CAD build for the part. Positions are in the model's coordinates, mm. A direction names the side the tool comes from. Give positions to 0.01 mm unless a question says otherwise; leave off trailing zeros. Write each loop counter-clockwise with the first axis right and the second up, starting at its lowest first coordinate (ties: lowest second). Pieces come first, ordered by that corner, then holes. Notation, with made-up numbers: (47, 58.5) -> (67, 58.5) arc R22 ccw to (67, 93.5) -> close; hole circle Ø4 at (-15.75, 6). An arc over 180 degrees is marked (long way). Answer as a JSON object with one key per item and string values.
```python
from build123d import *

# Parameters (mm, degrees)
IZIM1_W                     = 100
IZIM1_H                     = 100
Y_KSEKLIK_EKSTR_ZYON1_DEPTH = 8
IZIM2_W                     = 100
IZIM2_H                     = 100
Y_KSEKLIK_EKSTR_ZYON2_DEPTH = 30
IZIM3_W                     = 100
IZIM3_H                     = 100
KES_EKSTR_ZYON1_DEPTH       = 30


with BuildPart() as part:
    # Çizim1 → Yükseklik-Ekstrüzyon1 (new body)
    with BuildSketch(Plane(origin=(0, 0, 0), x_dir=(1, 0, 0), z_dir=(0, 1, 0))):
        with Locations((50, 50)):
            Rectangle(IZIM1_W, IZIM1_H)
    extrude(amount=Y_KSEKLIK_EKSTR_ZYON1_DEPTH)

    # Çizim2 → Yükseklik-Ekstrüzyon2 (add)
    with BuildSketch(Plane(origin=(0, 8, 0), x_dir=(1, 0, 0), z_dir=(0, 1, 0))):
        with Locations((50, 50)):
            Rectangle(IZIM2_W, IZIM2_H)
        Polygon((55, 28.75), (71.25, 28.75), (71.25, 71.25), (28.75, 71.25), (28.75, 28.75), (45, 28.75), (45, 20.75), (55, 20.75), align=None, mode=Mode.SUBTRACT)
    extrude(amount=Y_KSEKLIK_EKSTR_ZYON2_DEPTH)

    # Çizim3 → Kes-Ekstrüzyon1 (cut)
    with BuildSketch(Plane(origin=(0, 38, 0), x_dir=(1, 0, 0), z_dir=(0, 1, 0))):
        with Locations((50, 50)):
            Rectangle(IZIM3_W, IZIM3_H)
        Polygon((18.75, 81.25), (81.25, 81.25), (81.25, 18.75), (65, 18.75), (65, 10.75), (35, 10.75), (35, 18.75), (18.75, 18.75), align=None, mode=Mode.SUBTRACT)
    extrude(amount=-KES_EKSTR_ZYON1_DEPTH, mode=Mode.SUBTRACT)


solid = part.part
```
1) Slice it at C-C (x = 25.5). List the corners of the cut face in (y, z), then the cut area to 4 significant figures.
Model answer:
{"outline": "(0, -100) -> (8, -100) -> (8, -81.25) -> (38, -81.25) -> (38, -18.75) -> (8, -18.75) -> (8, 0) -> (0, 0) -> close", "area": "2,675 mm2"}
2) Slice it at B-B (z = -47). List the corners of the cut face in (x, y), then the cut area to 3 significant figures.
Model answer:
{"outline": "(0, 0) -> (100, 0) -> (100, 8) -> (81.25, 8) -> (81.25, 38) -> (71.25, 38) -> (71.25, 8) -> (28.75, 8) -> (28.75, 38) -> (18.75, 38) -> (18.75, 8) -> (0, 8) -> close", "area": "1,400 mm2"}
3) Slice it at A-A (y = 15). List the corners of the cut face in (x, z).
Model answer:
{"outline": "(18.75, -81.25) -> (81.25, -81.25) -> (81.25, -18.75) -> (65, -18.75) -> (65, -10.75) -> (35, -10.75) -> (35, -18.75) -> (18.75, -18.75) -> close; hole (28.75, -71.25) -> (71.25, -71.25) -> (71.25, -28.75) -> (55, -28.75) -> (55, -20.75) -> (45, -20.75) -> (45, -28.75) -> (28.75, -28.75) -> close"}
4) Mould opens along Z. For faces 1 (the flat face through (71.25, 23, -50)), 2 (the flat face through (27, 23, -18.75)), 3 (the flat face through (49, 8, -84)) say: released by +Z, released by -Z, zero draft, split by the parting line, or undercut.
Model answer:
{"face 1": "undercut", "face 2": "released by +Z", "face 3": "zero draft"}
5) Slice it at D-D (z = -79.5). List the corners of the cut face in (x, y).
Model answer:
{"outline": "(0, 0) -> (100, 0) -> (100, 8) -> (81.25, 8) -> (81.25, 38) -> (18.75, 38) -> (18.75, 8) -> (0, 8) -> close"}
6) Pin check, flat tips, straight feed: pin 1 (8 mm diameter, centred on x = 63, y = 25.5, fed in from -Z); pin 2 (4 mm diameter, centred on y = 11.5, z = -64, fed in from -X); pin 3 (13 mm diameter, centred on x = 24.5, y = 25.5, fed in from +Z). Stop position of each tip, or through.
Model answer:
{"pin 1": "stops at z = -81.25", "pin 2": "stops at x = 18.75", "pin 3": "stops at z = -18.75"}
7) Wall check: probe 1 along Z at (x, y) = (69, 32); probe 2 along X at (y, z) = (30, -70); probe 3 along Z at (x, y) = (60.5, 15). Give the ranges that are in metal, low to high.
Model answer:
{"probe 1": "z = -81.25 to -71.25, -28.75 to -18.75", "probe 2": "x = 18.75 to 28.75, 71.25 to 81.25", "probe 3": "z = -81.25 to -71.25, -28.75 to -10.75"}
8) 3-axis set-ups, long thin cutter, end or side, ignore diameter. For faces 4 (the flat face through (18.75, 23, -50)), 5 (the flat face through (73, 23, -18.75)), 6 (the flat face through (50, 23, -71.25)), 7 (the flat face through (50, 23, -10.75)): which of +Z, -Z, +X, -X, +Y, -Y reach the whole face in a straight line?
Model answer:
{"face 4": "+Z, -Z, -X, +Y", "face 5": "+Z, +X, +Y", "face 6": "+Y", "face 7": "+Z, +X, -X, +Y"}
